```python
from build123d import *

# Parameters (mm, degrees)
SKETCH1_W           = 20
SKETCH1_H           = 10
SKETCH1_R           = 2.1
BOSS_EXTRUDE1_DEPTH = 20
SKETCH2_R           = 2.1
CUT_EXTRUDE1_DEPTH  = 30


with BuildPart() as part:
    # Sketch1 → Boss-Extrude1 (new body)
    with BuildSketch(Plane.XY):
        with Locations((10, 5)):
            Rectangle(SKETCH1_W, SKETCH1_H)
        with Locations((4, 5)):
            Circle(SKETCH1_R, mode=Mode.SUBTRACT)
        with Locations((16, 5)):
            Circle(SKETCH1_R, mode=Mode.SUBTRACT)
    extrude(amount=BOSS_EXTRUDE1_DEPTH)

    # Sketch2 → Cut-Extrude1 (cut)
    with BuildSketch(Plane.XZ):
        with Locations((10, 15)):
            Circle(SKETCH2_R)
        with Locations((10, 5)):
            Circle(SKETCH2_R)
    extrude(amount=-CUT_EXTRUDE1_DEPTH, mode=Mode.SUBTRACT)


solid = part.part
```
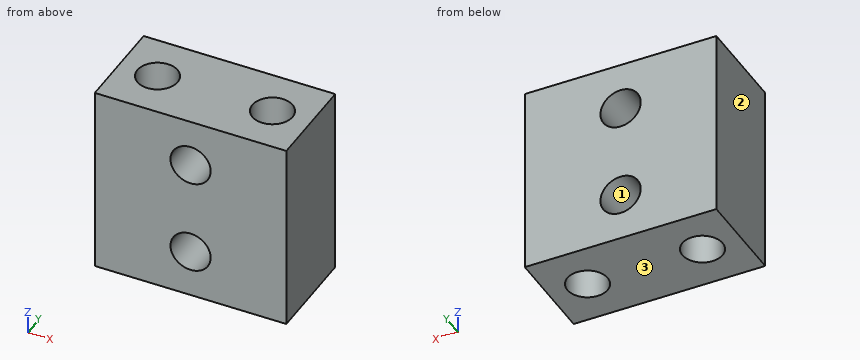
Check sheet for the modelled part. Datum: model origin and axes. Units: mm. Face numbers are marked on the shaded views. Round coordinates to 2 decimals unless told otherwise and drop trailing zeros. Write each loop counter-clockwise with the first axis right and the second up, starting at its lowest first coordinate (ties: lowest second). Pieces come first, ordered by that corner, then holes. Notation, with made-up numbers: (0.5, 10) -> (40.5, 10) arc R26 cw to (40.5, 27) -> close; hole circle Ø8 at (-18, 71.25). An arc over 180 degrees is marked (long way). Put each result on its own line as item: value.
(1) Sectioned sample at D-D (y = 7.5). Enter the section's corners in (x, z).
Values found:
outline: (0, 0) -> (20, 0) -> (20, 20) -> (0, 20) -> close; hole circle Ø4.2 at (10, 5); hole circle Ø4.2 at (10, 15)
(2) Sectioned sample at B-B (y = 5). Enter the section's corners in (x, z).
Values found:
outline: (0, 0) -> (1.9, 0) -> (1.9, 20) -> (0, 20) -> close; (6.1, 0) -> (13.9, 0) -> (13.9, 20) -> (6.1, 20) -> close; (18.1, 0) -> (20, 0) -> (20, 20) -> (18.1, 20) -> close; hole circle Ø4.2 at (10, 5); hole circle Ø4.2 at (10, 15)
(3) Mould release check, pull along X, two halves, no side actions. Record for the marked faces 1, 2 and 3: released by +X, released by -X, zero draft, split by the parting line, or undercut.
Values found:
face 1: undercut
face 2: released by -X
face 3: zero draft
(4) Sectioned sample at A-A (z = 5). Enter the section's corners in (x, y), plus the area to 3 significant figures.
Values found:
outline: (0, 0) -> (7.9, 0) -> (7.9, 10) -> (0, 10) -> close; (12.1, 0) -> (20, 0) -> (20, 10) -> (12.1, 10) -> close; hole circle Ø4.2 at (4, 5); hole circle Ø4.2 at (16, 5)
area: 130 mm^2
(5) Material ranges on line 1 (Z direction, x = 10, y = 8); line 2 (Z direction, x = 10.5, y = 3.75); line 3 (Y direction, x = 16, z = 4.5), recorded low to high.
Values found:
line 1: z = 0 to 2.9, 7.1 to 12.9, 17.1 to 20
line 2: z = 0 to 2.96, 7.04 to 12.96, 17.04 to 20
line 3: y = 0 to 2.9, 7.1 to 10
(6) Sectioned sample at C-C (x = 4). Enter the section's corners in (y, z), plus the area to 3 significant figures.
Values found:
outline: (0, 0) -> (2.9, 0) -> (2.9, 20) -> (0, 20) -> close; (7.1, 0) -> (10, 0) -> (10, 20) -> (7.1, 20) -> close
area: 116 mm^2
